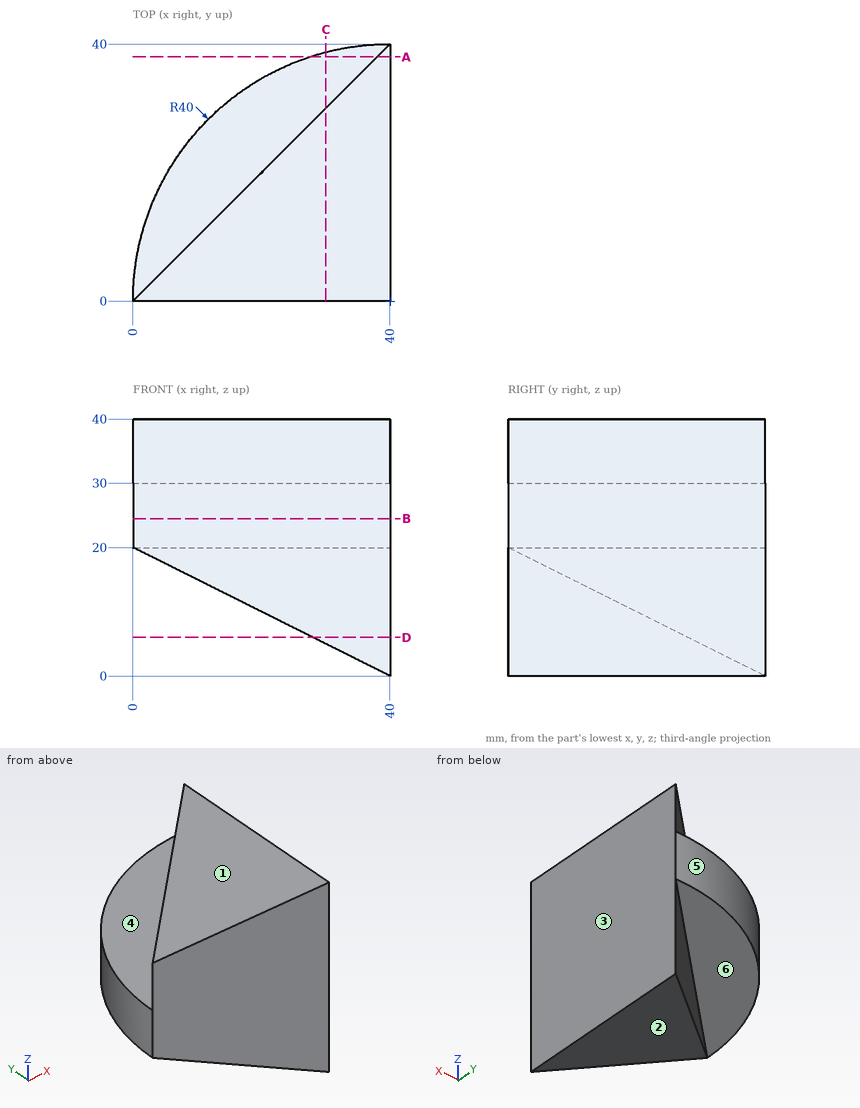
Part print with two shaded views. Sizes in mm from the minimum x, y, z corner. A direction names the side the tool comes from. Coordinates: 2 decimals unless noted, no trailing zeros. Write each loop counter-clockwise with the first axis right and the second up, starting at its lowest first coordinate (ties: lowest second). Pieces come first, ordered by that corner, then holes. Notation, with made-up numbers: (32.25, -39) - (66.25, -39) arc R8 cw to (66.25, -25) - close; hole circle Ø6 at (-6.5, 39). An arc over 180 degrees is marked (long way). Use a Markdown table: item, result. Add a question column.
Item 1: Drill centre lines: line 1 along Z through (x, y) = (10.5, 24.5); line 2 along Y through (x, z) = (25, 10.5); line 3 along Y through (x, z) = (20, 17). Where is each one in solid material? Low to high.
Item 2: Band-saw the part on D-D, the plane z = 6. Write the cut outline in (x, y).
Item 3: Band-saw the part on A-A, the plane y = 38. Write the cut outline in (x, z).
Item 4: 3-axis set-ups, long thin cutter, end or side, ignore diameter. For the marked faces 4, 5 and 6: which of +Z, -Z, +X, -X, +Y, -Y reach the whole face in a straight line?
Item 5: Drop flat-ended pins along their axis: pin 1 (4 mm diameter, centred on x = 20, y = 9, fed in from -Z); pin 2 (10 mm diameter, centred on x = 5.5, y = 26.5, fed in from +Z); pin 3 (1.5 mm diameter, centred on y = 34.5, z = 27, fed in from -X); pin 4 (6 mm diameter, centred on x = 8.5, z = 15.5, fed in from -Y). Give the stop position or say it passes through.
Item 6: Band-saw the part on B-B, the plane z = 24.5. Write the cut outline in (x, y).
Item 7: Two-plate mould, pull along X, no slides. Class the marked faces 1, 2 and 3: pulls with the +X half, pulls with the -X half, needs draft (parallel to the pull), parting line crosses it, or undercut.
Item 8: Band-saw the part on C-C, the plane x = 30. Write the cut outline in (y, z).
A:
| question | item | result |
|---|---|---|
| 1 | line 1 | z = 20 to 30 |
| 1 | line 2 | y = 0 to 25 |
| 1 | line 3 | y = 0 to 20 |
| 2 | outline | (28, 0) - (40, 0) - (40, 40) - (28, 28) - close |
| 3 | outline | (27.51, 20) - (38, 20) - (38, 1) - (40, 0) - (40, 40) - (38, 40) - (38, 30) - (27.51, 30) - close |
| 4 | face 4 | +Z, -X, +Y |
| 4 | face 5 | +Z, -Z, -X, +Y |
| 4 | face 6 | -Z, -X, +Y |
| 5 | pin 1 | stops at z = 9 |
| 5 | pin 2 | stops at z = 30 |
| 5 | pin 3 | stops at x = 18.53 |
| 5 | pin 4 | stops at y = 0 |
| 6 | outline | (0, 0) - (40, 0) - (40, 40) arc R40 ccw to start |
| 7 | face 1 | needs draft |
| 7 | face 2 | pulls with the -X half |
| 7 | face 3 | pulls with the +X half |
| 8 | outline | (0, 5) - (30, 5) - (30, 20) - (38.73, 20) - (38.73, 30) - (30, 30) - (30, 40) - (0, 40) - close |
